from build123d import *

# Parameters (mm, degrees)
SKETCH1_R           = 7.5
SKETCH1_R_2         = 25
BOSS_EXTRUDE1_DEPTH = 2
CUT_EXTRUDE1_REACH  = 145.192
SKETCH2_R           = 2
BOSS_EXTRUDE2_DEPTH = 2
SKETCH4_W           = 2
SKETCH4_H           = 6.5
SKETCH4_W_2         = 6.5
SKETCH4_H_2         = 2
BOSS_EXTRUDE3_DEPTH = 1


with BuildPart() as part:
    # Sketch1 → Boss-Extrude1 (new body)
    # profile 1 of 2: a face of its own
    with BuildSketch(Plane.XY):
        with BuildLine():
            ThreePointArc((-60, 0), (-52.867640737, 28.372743309), (-33.166247904, 50))
            Line((-33.166247904, 50), (-60, 50))
            Line((-60, 50), (-60, 0))
        make_face()
    # profile 2 of 2: a face of its own
    with BuildSketch(Plane.XY):
        with BuildLine():
            ThreePointArc((0, 60), (-17.320508076, 57.445626465), (-33.166247904, 50))
            ThreePointArc((-33.166247904, 50), (-52.867640737, 28.372743309), (-60, 0))
            ThreePointArc((-60, 0), (-6.678621673, -59.627141576), (58.513200418, -13.274237334))
            Line((58.513200418, -13.274237334), (99.152169538, -13.274237334))
            Line((99.152169538, -13.274237334), (121.213203436, 8.786796564))
            ThreePointArc((121.213203436, 8.786796564), (127.716385975, 41.480502971), (100, 60))
            Line((100, 60), (0, 60))
        make_face()
        Circle(SKETCH1_R, mode=Mode.SUBTRACT)
        with Locations((100, 30)):
            Circle(SKETCH1_R_2, mode=Mode.SUBTRACT)
    extrude(amount=BOSS_EXTRUDE1_DEPTH)

    # Sketch2 → Cut-Extrude1 (cut, up to next)
    with BuildSketch(Plane.XY.offset(2), mode=Mode.PRIVATE) as cut_extrude1_sk1:
        with Locations((55, 45)):
            Circle(SKETCH2_R)
    cut_extrude1_tool1 = extrude(cut_extrude1_sk1.sketch, amount=-CUT_EXTRUDE1_REACH, mode=Mode.PRIVATE) & part.part
    # Sketch2 → Cut-Extrude1 (cut, up to next)
    with BuildSketch(Plane.XY.offset(2), mode=Mode.PRIVATE) as cut_extrude1_sk2:
        with Locations((70, 11.725762666)):
            Circle(SKETCH2_R)
    cut_extrude1_tool2 = extrude(cut_extrude1_sk2.sketch, amount=-CUT_EXTRUDE1_REACH, mode=Mode.PRIVATE) & part.part
    add(cut_extrude1_tool1.solids().sort_by_distance((55, 45, 2))[0], mode=Mode.SUBTRACT)
    add(cut_extrude1_tool2.solids().sort_by_distance((70, 11.725763, 2))[0], mode=Mode.SUBTRACT)

    # Sketch3 → Boss-Extrude2 (add)
    with BuildSketch(Plane(origin=(0, 0, 0), x_dir=(-1, 0, 0), z_dir=(0, 0, -1))):
        with BuildLine():
            Line((-30, 80), (-30, 60))
            Line((-30, 60), (0, 60))
            ThreePointArc((0, 60), (2.502176759, 59.947803225), (5, 59.791303715))
            Line((5, 59.791303715), (5, 80))
            Line((5, 80), (-30, 80))
        make_face()
    extrude(amount=-BOSS_EXTRUDE2_DEPTH)

    # Sketch4 → Boss-Extrude3 (add)
    with BuildSketch(Plane(origin=(0, 0, 0), x_dir=(-1, 0, 0), z_dir=(0, 0, -1))):
        with Locations((-12.5, 68.846087829)):
            Rectangle(SKETCH4_W, SKETCH4_H)
        with Locations((-16.75, 64.596087829)):
            Rectangle(SKETCH4_W_2, SKETCH4_H_2)
        with Locations((-12.5, 64.596087829)):
            Rectangle(SKETCH4_W, SKETCH4_H_2)
        with Locations((-8.25, 64.596087829)):
            Rectangle(SKETCH4_W_2, SKETCH4_H_2)
        with Locations((-12.5, 60.346087829)):
            Rectangle(SKETCH4_W, SKETCH4_H)
    extrude(amount=BOSS_EXTRUDE3_DEPTH)


solid = part.part
Design review of the part built by this model. Coordinates are the model's own, in mm. Give positions to 0.01 mm unless a question says otherwise; leave off trailing zeros. Loops run counter-clockwise (first coordinate to the right, second up) from the corner with the lowest first, then second, coordinate; pieces in that order, holes last. Notation, with made-up numbers: (-11.5, -14.75) -> (0.5, -14.75) arc R21 ccw to (0.5, -3.75) -> close; hole circle Ø5 at (79.5, 53). An arc over 180 degrees is marked (long way). One line per question, with ' | ' between items. Start each with the question number.
(1) Insertion check: P1, Ø8, axis at x = 9.5, y = 35.5, coming from the -Z side; P2, Ø1.6, axis at x = -52, z = 1, coming from the +Y side; P3, Ø0.5, axis at x = 15.5, z = -0.5, coming from the +Y side; P4, Ø9, axis at x = 0, y = 0, coming from the +Z side. Each pin has a flat end and moves straight along its axis. Give the tip position at first contact, or say it passes through.
(2) We need section D-D (z = 0.45). State the section outline as (x, y) points.
(3) Draft analysis for pull direction Y (two halves, no side actions). For faces 1 (the face through (71.908, 12.327, 1.014)), 2 (the face through (15, 11, 0)), 3 (the face through (127.902, 41.022, 0.986)), state which applies: +Y half, -Y half, draft (parallel to the pull), parting line (faces both ways), or undercut.
(4) We need section A-A (x = 70). State the section outline as (y, z) points, and give its area (3 significant figures).
(5) For line 1 (Y direction, x = 0, z = 1.15); line 2 (Z direction, x = -34, y = -44); line 3 (Y direction, x = 55, z = 0.5), list the stretches that pass through material, from the lowest coordinate up.
(6) We need section B-B (y = 30). State the section outline as (x, z) points.
(7) We need section C-C (y = 45). State the section outline as (x, z) points, and give its area (3 significant figures).
The answers:
1) P1: stops at z = 0 | P2: stops at y = 50 | P3: stops at y = 65.6 | P4: passes through
2) outline: (-60, 0) arc R60 ccw to (58.51, -13.27) -> (99.15, -13.27) -> (121.21, 8.79) arc R30 ccw to (100, 60) -> (30, 60) -> (30, 80) -> (-5, 80) -> (-5, 59.79) arc R60 ccw to (-33.17, 50) -> (-60, 50) -> close; hole circle Ø15 at (0, 0); hole circle Ø4 at (55, 45); hole circle Ø4 at (70, 11.73); hole circle Ø50 at (100, 30)
3) face 1: undercut | face 2: draft | face 3: parting line
4) outline: (-13.27, 0) -> (9.73, 0) -> (9.73, 2) -> (-13.27, 2) -> close; (13.73, 0) -> (60, 0) -> (60, 2) -> (13.73, 2) -> close | area: 139 mm^2
5) line 1: y = -60 to -7.5, 7.5 to 80 | line 2: z = 0 to 2 | line 3: y = -23.98 to 43, 47 to 60
6) outline: (-60, 0) -> (75, 0) -> (75, 2) -> (-60, 2) -> close; (125, 0) -> (130, 0) -> (130, 2) -> (125, 2) -> close
7) outline: (-60, 0) -> (53, 0) -> (53, 2) -> (-60, 2) -> close; (57, 0) -> (80, 0) -> (80, 2) -> (57, 2) -> close; (120, 0) -> (125.98, 0) -> (125.98, 2) -> (120, 2) -> close | area: 284 mm^2
